Verification items for the finished model (mm, model axes). Face numbers are marked on the shaded views. A direction names the side the tool comes from. Coordinates: 2 decimals unless noted, no trailing zeros. Write each loop counter-clockwise with the first axis right and the second up, starting at its lowest first coordinate (ties: lowest second). Pieces come first, ordered by that corner, then holes. Notation, with made-up numbers: (3, 78) - (8, 78) arc R6 cw to (8, 85) - close; hole circle Ø2 at (-33, 44.25). An arc over 180 degrees is marked (long way). Answer as CSV lines item,"result". Start each with the question number.
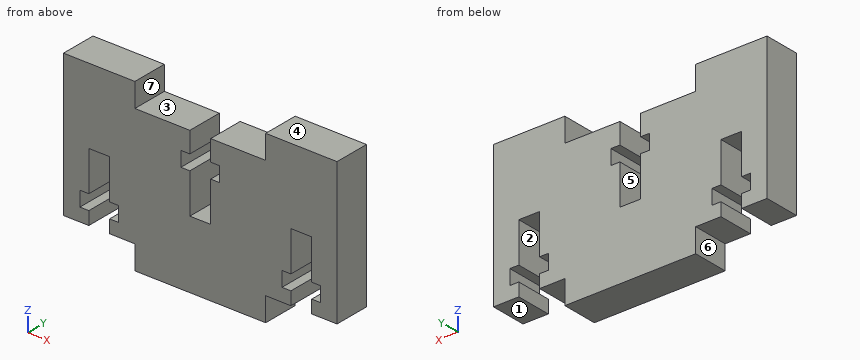
Autodesk Inventor part; units mm, degrees
ref_plane "РабПлоскость2" through (57.5, -97.5, 20) normal (0, 0, -1) x (0, 1, 0)
ref_plane "YZ Plane" through (0, 0, 0) normal (1, 0, 0) x (0, 1, 0)
ref_plane "XZ Plane" through (0, 0, 0) normal (0, 1, 0) x (-1, 0, 0)
ref_plane "РабПлоскость1" through (0, 0, 0) normal (0, 0, 1) x (1, 0, 0)
sketch "Эскиз1" plane through (0, 0, 0) normal (0, 0, 1) x (1, 0, 0)
  line L0 (111.5, 97.5) -> (111.5, -97.5)
  line L1 (65.5, 97.5) -> (111.5, 97.5)
  line L2 (65.5, 63.1836) -> (65.5, 97.5)
  line L3 (65.5, 63.1836) -> (57.5, 63.1836)
  line L4 (57.5, 53.1836) -> (57.5, 63.1836)
  line L5 (65.5, 53.1836) -> (57.5, 53.1836)
  line L6 (65.5, -53.1539) -> (65.5, 53.1836)
  line L7 (65.5, -53.1539) -> (57.5, -53.1539)
  line L8 (57.5, -63.1539) -> (57.5, -53.1539)
  line L9 (65.5, -63.1539) -> (57.5, -63.1539)
  line L10 (65.5, -97.5) -> (65.5, -63.1539)
  line L11 (111.5, -97.5) -> (65.5, -97.5)
  line L12 (65.5, 53.1836) -> (111.5, 53.1836)
  line L13 (111.5, 53.1836) -> (111.5, 47.1836)
  line L14 (111.5, 47.1836) -> (65.5, 47.1836)
  line L15 (65.5, 47.1836) -> (65.5, 53.1836)
  line L16 (65.5, -53.1539) -> (111.5, -53.1539)
  line L17 (111.5, -53.1539) -> (111.5, -47.1539)
  line L18 (111.5, -47.1539) -> (65.5, -47.1539)
  line L19 (65.5, -47.1539) -> (65.5, -53.1539)
  point P0 (0, 0)
  dimension "d0" = 6
  dimension "d1" = 6
ref_plane "РабПлоскость2" through (57.5, -97.5, 20) normal (0, 0, -1) x (0, 1, 0)
extrude "Выдавливание1" add sketch "Эскиз1" along normal up to surface (20 mm away) contours L0 L16 L6 L18
sketch "Эскиз2" plane through (65.5, -53.1539, 0) normal (0, -1, 0) x (1, 0, 0)
  line L0 (46, 24) -> (0, 24)
  line L1 (0, 20) -> (46, 20)
  line L2 (0, 20) -> (12, 20)
  line L3 (12, 20) -> (12, 24)
  line L4 (12, 24) -> (0, 24)
  line L5 (0, 24) -> (0, 20)
  line L6 (46, 20) -> (34, 20)
  line L7 (34, 20) -> (34, 24)
  line L8 (34, 24) -> (46, 24)
  line L9 (46, 24) -> (46, 20)
  point P0 (-65.5, 0)
  point P1 (34, 20)
  dimension "d4" = 12
  dimension "d5" = 12
sketch "Эскиз3" plane through (65.5, -53.1539, 0) normal (0, -1, 0) x (1, 0, 0)
  line L0 (31, 10.1574) -> (31, 5.1574)
  line L1 (26.25, 14.0145) -> (19.75, 14.0145)
  line L2 (19.75, 14.0145) -> (19.75, 16.5145)
  line L3 (19.75, 16.5145) -> (26.25, 16.5145)
  line L4 (26.25, 16.5145) -> (26.25, 14.0145)
  line L5 (24.75, 20) -> (21.25, 20)
  line L6 (21.25, 20) -> (21.25, 7.3147)
  line L7 (21.25, 7.3147) -> (24.75, 7.3147)
  line L8 (24.75, 7.3147) -> (24.75, 20)
  line L9 (24.75, 20) -> (21.25, 7.3147) construction
  line L10 (21.25, 20) -> (24.75, 7.3147) construction
  line L11 (24.75, 20) -> (21.25, 16.5145)
  line L12 (24.75, 16.5145) -> (21.25, 20)
  line L13 (46, 20) -> (0, 20)
  point P0 (-65.5, 0)
  point P1 (23, 13.6574)
  point P2 (23, 20)
  point P3 (21.25, 14.0145)
  point P4 (24.75, 14.0145)
  dimension "d6" = 6.5
  dimension "d7" = 2.5
  dimension "d10" = 4.75
  dimension "d12" = 3.5
  dimension "d13" = 3.25
extrude "Выдавливание2" add sketch "Эскиз2" against normal blind 6 contours L9 L1 L7 L0 | L3 L1 L5 L0
extrude "Выдавливание3" cut sketch "Эскиз3" against normal blind 6
sketch "Эскиз4" plane through (65.5, -53.1539, 0) normal (0, -1, 0) x (1, 0, 0)
  line L0 (46, 0) -> (0, 0)
  line L1 (12, 0) -> (34, 0)
  line L2 (34, 0) -> (34, -4)
  line L3 (34, -4) -> (12, -4)
  line L4 (12, -4) -> (12, 0)
  point P0 (-65.5, 0)
  point P1 (34, 0)
  dimension "d18" = 12
  dimension "d19" = 12
  dimension "d20" = 4
extrude "Выдавливание4" add sketch "Эскиз4" against normal blind 6
sketch "Эскиз5" plane through (65.5, -53.1539, 24) normal (0, -1, 0) x (1, 0, 0)
  line L0 (9.25, -21.8) -> (2.75, -21.8)
  line L1 (2.75, -21.8) -> (2.75, -19.3)
  line L2 (2.75, -19.3) -> (9.25, -19.3)
  line L3 (9.25, -19.3) -> (9.25, -21.8)
  line L4 (4.25, -12.6005) -> (7.75, -12.6005)
  line L5 (7.75, -12.6005) -> (7.75, -24)
  line L6 (7.75, -24) -> (4.25, -24)
  line L7 (4.25, -24) -> (4.25, -12.6005)
  line L8 (4.25, -12.6005) -> (7.75, -24) construction
  line L9 (7.75, -12.6005) -> (4.25, -24) construction
  line L10 (0, -24) -> (12, -24)
  line L11 (43.25, -19.3) -> (43.25, -21.8)
  line L12 (41.75, -24) -> (38.25, -24)
  line L13 (41.75, -12.6) -> (41.75, -24)
  line L14 (43.25, -21.8) -> (36.75, -21.8)
  line L15 (36.75, -19.3) -> (43.25, -19.3)
  line L16 (38.25, -12.6) -> (41.75, -24) construction
  line L17 (38.25, -12.6) -> (41.75, -12.6)
  line L18 (41.75, -12.6) -> (38.25, -24) construction
  line L19 (36.75, -21.8) -> (36.75, -19.3)
  line L20 (38.25, -24) -> (38.25, -12.6)
  line L21 (34, -24) -> (46, -24)
  point P0 (-65.5, -24)
  point P1 (6, -18.3002)
  point P2 (6, -24)
  point P3 (40, -18.3)
  point P4 (42.6795, -22.1366)
  point P5 (40, -24)
  point P6 (38.25, -19.3)
  point P7 (38.25, -21.8)
  point P8 (41.75, -21.8)
  point P9 (41.75, -19.3)
  point P10 (4.25, -19.3)
  point P11 (4.25, -21.8)
  point P12 (7.75, -21.8)
  point P13 (7.75, -19.3)
  dimension "d23" = 6.5
  dimension "d24" = 2.5
  dimension "d29" = 3.5
  dimension "d30" = 3.25
  dimension "d31" = 2.2
  dimension "d32" = 6.5
  dimension "d33" = 2.5
  dimension "d34" = 3.5
  dimension "d35" = 3.25
  dimension "d36" = 2.2
  dimension "d39" = 6.7
extrude "Выдавливание5" cut sketch "Эскиз5" against normal blind 6
properties part number "стенка держит стенку"
1. Cross-section at D-D (x = 81.5). Record the cut outline in (y, z).
2. Cross-section at C-C (z = 3.25). Record the cut outline in (x, y).
3. Scan lines: line 1 along X through (y, z) = (-51.5, 6); line 2 along X through (y, z) = (-51, 10.5); line 3 along Z through (x, y) = (91.5, -47.5). Record each from-to range of solid material in increasing order. Write a range as from..to.
4. Draft check along X on the marked faces 4, 5, 6 and 7. Enter one of: pulls with the +X half, pulls with the -X half, needs draft (parallel to the pull), parting line crosses it, or undercut.
5. Cross-section at A-A (z = 17.25). Record the cut outline in (x, y), and give its area (3 significant figures).
6. Access from +Z, -Z, +X, -X, +Y, -Y to the whole of each face (thin tool, end or side, straight path). Record for the marked faces 1, 2 and 3.
7. Depth check by flat-ended pin: P1, Ø2, axis at x = 68, y = -51.5, coming from the -Z side; P2, Ø1, axis at x = 96, y = -51, coming from the +Z side; P3, Ø2, axis at y = -51, z = -2.5, coming from the -X side. Enter the tip coordinate at first touch or a pass-through.
8. Cross-section at B-B (x = 69). Record the cut outline in (y, z), and give its area (3 significant figures).
Completed:
1,outline,"(-53.15, -4) - (-47.15, -4) - (-47.15, 20) - (-53.15, 20) - close"
2,outline,"(65.5, -53.15) - (68.25, -53.15) - (68.25, -47.15) - (65.5, -47.15) - close; (74.75, -53.15) - (102.25, -53.15) - (102.25, -47.15) - (74.75, -47.15) - close; (108.75, -53.15) - (111.5, -53.15) - (111.5, -47.15) - (108.75, -47.15) - close"
3,line 1,"x = 65.5..69.75, 73.25..103.75, 107.25..111.5"
3,line 2,"x = 65.5..69.75, 73.25..86.75, 90.25..103.75, 107.25..111.5"
3,line 3,"z = -4..14.01, 16.51..20"
4,face 4,"needs draft"
4,face 5,"undercut"
4,face 6,"pulls with the -X half"
4,face 7,"undercut"
5,outline,"(65.5, -53.15) - (86.75, -53.15) - (86.75, -47.15) - (65.5, -47.15) - close; (90.25, -53.15) - (111.5, -53.15) - (111.5, -47.15) - (90.25, -47.15) - close"
5,area,"255 mm2"
6,face 1,"-Z, +X, +Y, -Y"
6,face 2,"-Z, +Y, -Y"
6,face 3,"+Z, +Y, -Y"
7,P1,"stops at z = 0"
7,P2,"stops at z = 20"
7,P3,"stops at x = 77.5"
8,outline,"(-53.15, 0) - (-47.15, 0) - (-47.15, 2.2) - (-53.15, 2.2) - close; (-53.15, 4.7) - (-47.15, 4.7) - (-47.15, 24) - (-53.15, 24) - close"
8,area,"129 mm2"
